Geometry check sheet. Reference: drawing and pictorial views, mm from the part's lowest x, y, z. A direction names the side the tool comes from. Give positions to 0.01 mm unless a question says otherwise; leave off trailing zeros. Loops run counter-clockwise (first coordinate to the right, second up) from the corner with the lowest first, then second, coordinate; pieces in that order, holes last. Notation, with made-up numbers: (21, -10) -> (50, -10) arc R9 ccw to (50, -1) -> close; hole circle Ø3 at (20.5, 42.25). An arc over 180 degrees is marked (long way). Write each question's results on one line, items separated by ' | '. Start each with the question number.
1. Mould release check, pull along Z, two halves, no side actions. Record for the marked faces 1, 2, 3 and 4: +Z half, -Z half, draft (parallel to the pull), parting line (faces both ways), or undercut.
2. Material ranges on L1, parallel to X at y = 3.25, z = 15.5 (1 decimal); L2, parallel to X at y = 11.5, z = 12.5 (1 decimal); L3, parallel to Y at x = 6.5, z = 6.75, recorded low to high. Write a range as from..to.
3. Cross-section at D-D on y = 3. Record the boundary of the cut face in (x, z) (1 decimal), and give its area (3 significant figures).
4. Cross-section at C-C on y = 11.75. Record the boundary of the cut face in (x, z) (1 decimal), and give its area (3 significant figures).
5. Cross-section at B-B on z = 12.5. Record the boundary of the cut face in (x, y) (1 decimal).
6. Gauge pin test, flat ends, axial feed: pin 1 Ø5.5 at (y, z) = (14.5, 14) entering from +X; pin 2 Ø2.5 at (y, z) = (2.5, 10.5) entering from -X; pin 3 Ø6 at (x, z) = (9.5, 13.5) entering from -Y; pin 4 Ø1.8 at (x, z) = (6.6, 12.5) entering from -Y. Record the tip position at first contact, or that the pin passes through.
7. Tool access check on the marked faces 5, 6 and 7. Record the directions out of +Z, -Z, +X, -X, +Y, -Y that give a thin tool (end or side, any length) a straight path to the whole face; none if there is none.
8. Cross-section at A-A on y = 7. Record the boundary of the cut face in (x, z) (1 decimal), and give its area (3 significant figures).
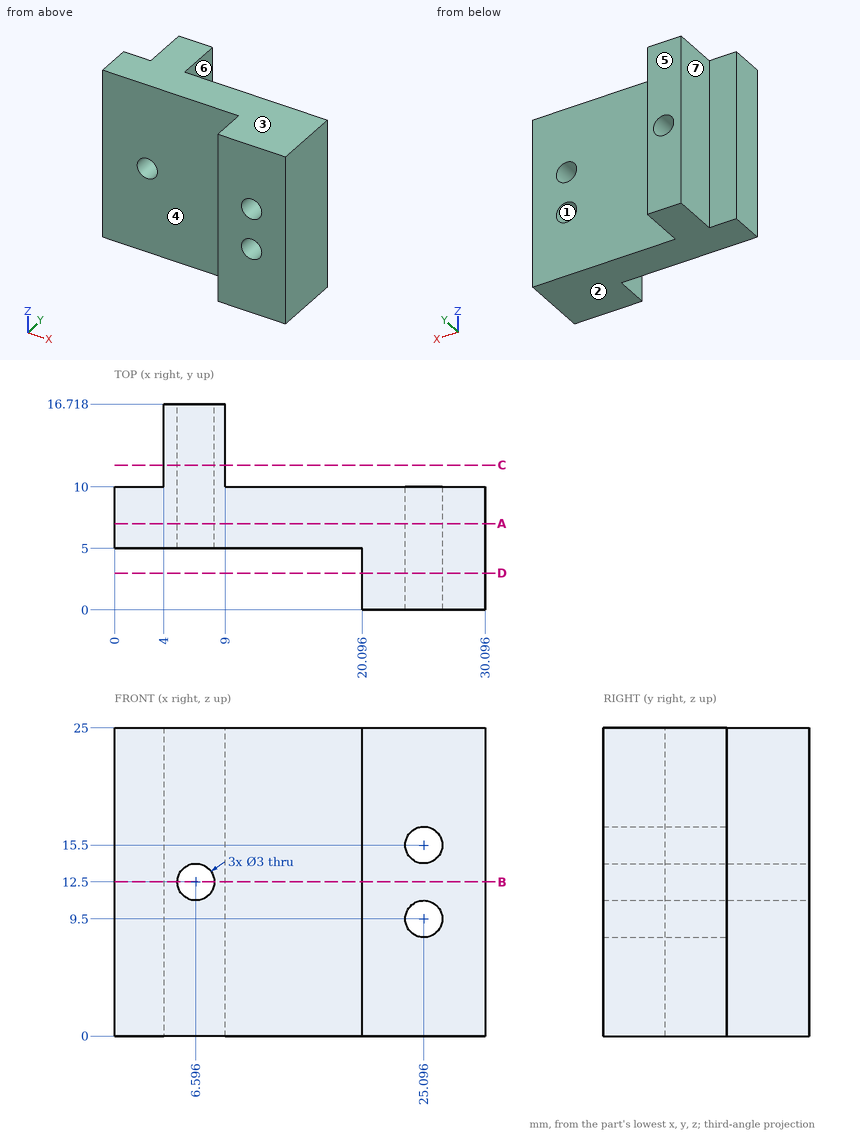
Geometry says:
1) face 1: undercut | face 2: -Z half | face 3: +Z half | face 4: draft
2) L1: 20.1..23.6, 26.6..30.1 | L2: 4..5.1, 8.1..9 | L3: 5..16.72
3) outline: (20.1, 0) -> (30.1, 0) -> (30.1, 25) -> (20.1, 25) -> close; hole circle Ø3 at (25.1, 9.5); hole circle Ø3 at (25.1, 15.5) | area: 236 mm^2
4) outline: (4, 0) -> (9, 0) -> (9, 25) -> (4, 25) -> close; hole circle Ø3 at (6.6, 12.5) | area: 118 mm^2
5) outline: (0, 5) -> (5.1, 5) -> (5.1, 16.7) -> (4, 16.7) -> (4, 10) -> (0, 10) -> close; (8.1, 5) -> (20.1, 5) -> (20.1, 0) -> (30.1, 0) -> (30.1, 10) -> (9, 10) -> (9, 16.7) -> (8.1, 16.7) -> close
6) pin 1: x = 9 | pin 2: x = 20.1 | pin 3: y = 5 | pin 4: through
7) face 5: +Z, -Z, +X, -X, +Y | face 6: +Z, -Z, +X, +Y | face 7: +Z, -Z, -X, +Y
8) outline: (0, 0) -> (30.1, 0) -> (30.1, 25) -> (0, 25) -> close; hole circle Ø3 at (6.6, 12.5); hole circle Ø3 at (25.1, 9.5); hole circle Ø3 at (25.1, 15.5) | area: 731 mm^2
